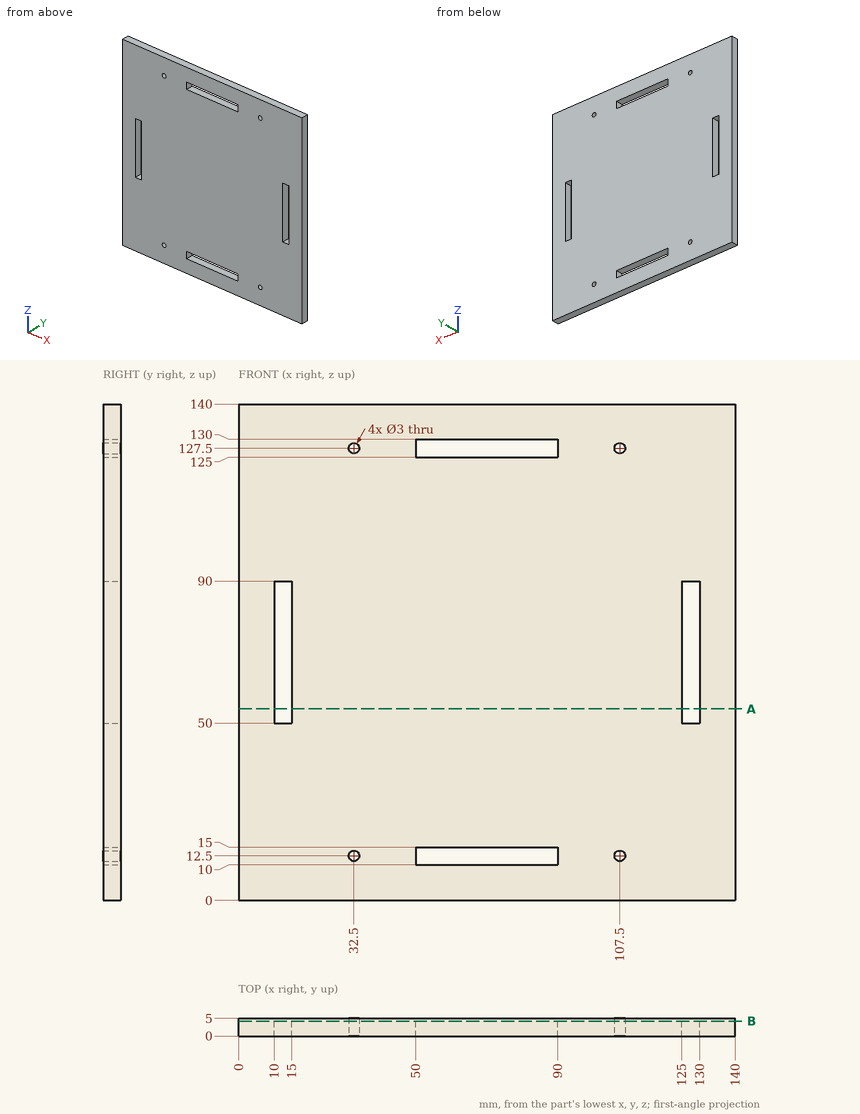
Could you check a few things on this drawing? It's one solid part, dimensions in mm from its lowest x, y, z. Coordinates: 2 decimals unless noted, no trailing zeros. Order: outer loops, then holes, each group sorted by start corner. A loop starts at its lowest first (then second) coordinate and runs counter-clockwise, first axis right, second up.
1. I need wall thicknesses on line 1 (Z direction, x = 32.5, y = 2.35); line 2 (X direction, y = 3.85, z = 12.5); line 3 (X direction, y = 2.85, z = 76). Which ranges of each line are inside material? Lowest first, please.
2. If we section it at A-A (z = 54): Please give me the cut outline in (x, y).
3. If we section it at B-B (y = 4.2): Give the number of separate pieces and of enclosed holes in the cut face, then the cut area to 3 significant figures.
Entries:
1. line 1: z = 0 to 11, 14 to 126, 129 to 140
1. line 2: x = 0 to 31, 34 to 50, 90 to 106, 109 to 140
1. line 3: x = 0 to 10, 15 to 125, 130 to 140
2. outline: (0, 0) - (10, 0) - (10, 5) - (0, 5) - close; (15, 0) - (125, 0) - (125, 5) - (15, 5) - close; (130, 0) - (140, 0) - (140, 5) - (130, 5) - close
3. separate pieces: 1
3. enclosed holes: 8
3. area: 18,800 mm2
